Source: CAD feature listing. Evaluate the final solid. Frame: model axes, mm. A direction names the side the tool comes from. Coordinates: 2 decimals unless noted, no trailing zeros. Loops run counter-clockwise (first coordinate to the right, second up) from the corner with the lowest first, then second, coordinate; pieces in that order, holes last. Notation, with made-up numbers: (75.5, -9) - (95.5, -9) arc R10 cw to (95.5, -1) - close; hole circle Ø11 at (88, -24.75). An arc over 180 degrees is marked (long way). Use CSV: the item, a comma, the result in double quotes. Start each with the question number.
```python
from build123d import *

# Parameters (mm, degrees)
F1_DEPTH = 25.4
F2_W     = 14.229968
F2_H     = 10.471108
F3_DEPTH = 14.424406


with BuildPart() as f1:
    # F0 (on Front) → F1 (new body, symmetric)
    with BuildSketch(Plane.XZ):
        Polygon((-36.380388, 23.492869), (-36.380388, -24.298338), (34.500958, -24.298338), (34.500958, 23.492869), (20.27099, 23.492869), (20.27099, -11.679313), (-22.15042, -11.679313), (-22.15042, 23.492869), align=None)
    extrude(amount=F1_DEPTH, both=True)

    # F2 (on face) → F3 (cut)
    with BuildSketch(Plane.XY.offset(23.492869)):
        with Locations((27.385974, 0.26849)):
            Rectangle(F2_W, F2_H)
    extrude(amount=-F3_DEPTH, mode=Mode.SUBTRACT)


solid = f1.part
```
(1) Section A-A on z = 17. Output: boundary loops of the cut face in (x, y).
(2) Pin query (flat end, axial travel): pin 1 Ø3 at (x, y) = (29, 1.5) entering from +Z; pin 2 Ø4 at (x, y) = (4, 18.5) entering from +Z; pin 3 Ø3 at (x, y) = (19, 7.5) entering from +Z. Return the tip coordinate at first contact, or that it passes through.
(3) Ray query, line 1 (X direction, y = 8, z = 15.5); line 2 (Y direction, x = 30.5, z = 18); line 3 (Z direction, x = 14, y = 6). Return the intervals inside material, ascending. Write a range as [from, to].
(4) Reachability of faces 1 (the flat face through (-1, 0, -11.679)), 2 (the flat face through (27, 5.504, 16)), 3 (the flat face through (27, 15, 23.493)) from +Z, -Z, +X, -X, +Y, -Y: full face, straight path, thin tool, end or side. Return the list, or none.
(5) Section C-C on y = -4. Output: boundary loops of the cut face in (x, z).
(6) Section B-B on z = 5.5. Output: boundary loops of the cut face in (x, y), plus the area to 3 significant figures.
(7) Draft query along Y for faces 4 (the flat face through (-1, -25.4, -16)), 5 (the flat face through (-36.38, 0, 0)), 6 (the flat face through (27, -4.967, 16)), 7 (the flat face through (-1, 25.4, -16)). Return one class per face: released by +Y, released by -Y, zero draft, split by the parting line, or undercut.
(8) Section D-D on x = -7. Output: boundary loops of the cut face in (y, z).
Solution:
1,outline,"(-36.38, -25.4) - (-22.15, -25.4) - (-22.15, 25.4) - (-36.38, 25.4) - close; (20.27, -25.4) - (34.5, -25.4) - (34.5, -4.97) - (20.27, -4.97) - close; (20.27, 5.5) - (34.5, 5.5) - (34.5, 25.4) - (20.27, 25.4) - close"
2,pin 1,"stops at z = 9.07"
2,pin 2,"stops at z = -11.68"
2,pin 3,"stops at z = 23.49"
3,line 1,"x = [-36.38, -22.15], [20.27, 34.5]"
3,line 2,"y = [-25.4, -4.97], [5.5, 25.4]"
3,line 3,"z = [-24.3, -11.68]"
4,face 1,"+Z, +Y, -Y"
4,face 2,"+Z, +X"
4,face 3,"+Z, +X, -X, +Y, -Y"
5,outline,"(-36.38, -24.3) - (34.5, -24.3) - (34.5, 9.07) - (20.27, 9.07) - (20.27, -11.68) - (-22.15, -11.68) - (-22.15, 23.49) - (-36.38, 23.49) - close"
6,outline,"(-36.38, -25.4) - (-22.15, -25.4) - (-22.15, 25.4) - (-36.38, 25.4) - close; (20.27, -25.4) - (34.5, -25.4) - (34.5, 25.4) - (20.27, 25.4) - close"
6,area,"1,450 mm²"
7,face 4,"released by -Y"
7,face 5,"zero draft"
7,face 6,"undercut"
7,face 7,"released by +Y"
8,outline,"(-25.4, -24.3) - (25.4, -24.3) - (25.4, -11.68) - (-25.4, -11.68) - close"
